The listing builds one solid part. Answer for the finished solid, in the listing's coordinates (mm). A direction names the side the tool comes from. Coordinates: 2 decimals unless noted, no trailing zeros. Order: outer loops, then holes, each group sorted by start corner. A loop starts at its lowest first (then second) coordinate and runs counter-clockwise, first axis right, second up. Notation, with made-up numbers: (78.5, 38.25) -> (108.5, 38.25) arc R20 ccw to (108.5, 59.25) -> close; hole circle Ø3 at (5, -29). An arc over 180 degrees is marked (long way). Return JSON: item names as keys, results as strings.
```python
from build123d import *

# Parameters (mm, degrees)
SKETCH1_W           = 150
SKETCH1_H           = 70
BOSS_EXTRUDE1_DEPTH = 10
SKETCH2_W           = 150
SKETCH2_H           = 3
BOSS_EXTRUDE2_DEPTH = 20
SKETCH3_W           = 110
SKETCH3_H           = 20
CUT_EXTRUDE1_DEPTH  = 105.947605976
FILLET1_R           = 5
FILLET2_R           = 10
FILLET3_R           = 2.5


with BuildPart() as part:
    # Sketch1 → Boss-Extrude1 (new body)
    with BuildSketch(Plane.XY):
        Rectangle(SKETCH1_W, SKETCH1_H)
        Polygon((-60, 25), (-55, 25), (55, 25), (60, 25), (60, 20), (55, 20), (55, -25), (-55, -25), (-55, 20), (-60, 20), align=None, mode=Mode.SUBTRACT)
    extrude(amount=BOSS_EXTRUDE1_DEPTH)

    # Sketch2 → Boss-Extrude2 (add)
    with BuildSketch(Plane.XY.offset(10)):
        with Locations((0, -33.5)):
            Rectangle(SKETCH2_W, SKETCH2_H)
    extrude(amount=BOSS_EXTRUDE2_DEPTH)

    # Sketch3 → Cut-Extrude1 (cut, through all)
    with BuildSketch(Plane(origin=(0, -32, 0), x_dir=(1, 0, 0), z_dir=(0, 1, 0))):
        with Locations((0, -20)):
            Rectangle(SKETCH3_W, SKETCH3_H)
    extrude(amount=-CUT_EXTRUDE1_DEPTH, mode=Mode.SUBTRACT)

    # Fillet1
    fillet1_edges = [part.edges().sort_by_distance(p)[0] for p in [
        (0, 25, 10),
        (0, -25, 10),
        (75, 1.5, 10),
        (0, 35, 10),
        (-75, 1.5, 10),
    ]]
    fillet(fillet1_edges, radius=FILLET1_R - 0.0001)  # a hair under: the kernel refuses the full size

    # Fillet2
    fillet2_edges = [part.edges().sort_by_distance(p)[0] for p in [
        (55, -33.5, 10),
        (-55, -33.5, 10),
    ]]
    fillet(fillet2_edges, radius=FILLET2_R)

    # Fillet3
    fillet3_edges = [part.edges().sort_by_distance(p)[0] for p in [
        (55, -4.99995, 10),
        (-55, -4.99995, 10),
        (-75, -33.5, 30),
        (75, -33.5, 30),
        (55, -33.5, 30),
        (-55, -33.5, 30),
    ]]
    fillet(fillet3_edges, radius=FILLET3_R)


solid = part.part
```
Item 1: Which of the six approach directions +Z, -Z, +X, -X, +Y, -Y give full straight-line access (tool end or side, diameter ignored) to faces 1 (the flat face through (55, -33, 24)), 2 (the flat face through (-1, -31, 0)), 3 (the cylindrical face through (73, 2, 9)), 4 (the flat face through (60, 23, 5)), 5 (the flat face through (-1, 25, 2))?
Answer list:
{"face 1": "+Z, +Y, -Y", "face 2": "-Z, +X, -X, +Y, -Y", "face 3": "+Z, +X, +Y", "face 4": "+Z", "face 5": "+Z, -Z"}
Item 2: Flat-ended cylindrical pins translate along their axes: pin 1 (6 mm diameter, centred on x = -7, z = 13.5, fed in from -Y); pin 2 (8 mm diameter, centred on x = 3, y = -24, fed in from +Z); pin 3 (3 mm diameter, centred on y = 24.5, z = 7.5, fed in from -X); pin 4 (6 mm diameter, centred on y = 15.5, z = 10, fed in from +X). Find the tip coordinate at first contact, or state that the pin passes through.
Answer list:
{"pin 1": "through", "pin 2": "z = 9.58", "pin 3": "x = -74.9", "pin 4": "x = 74.58"}
Item 3: The part is cut by section C-C on z = 15. Determine the outline of the cut face in (x, y).
Answer list:
{"outline": "(-75, -35) -> (-53.66, -35) -> (-53.66, -32) -> (-75, -32) -> close; (53.66, -35) -> (75, -35) -> (75, -32) -> (53.66, -32) -> close"}
Item 4: Find the intervals of material crossed by probe 1 along Y at (x, z) = (47, 2.5); probe 2 along Y at (x, z) = (-61, 12.5); probe 3 along Y at (x, z) = (-41.5, 7.75), in increasing order.
Answer list:
{"probe 1": "-35 to -25, 25 to 35", "probe 2": "-35 to -32", "probe 3": "-35 to -25.82, 25.82 to 34.18"}
Item 5: The part is cut by section D-D on z = 2. Determine the outline of the cut face in (x, y), plus the area to 3 significant figures.
Answer list:
{"outline": "(-75, -35) -> (75, -35) -> (75, 35) -> (-75, 35) -> close; hole (-60, 20) -> (-55, 20) -> (-55, -25) -> (55, -25) -> (55, 20) -> (60, 20) -> (60, 25) -> (-60, 25) -> close", "area": "4,950 mm2"}
Item 6: Determine the mould class of faces 6 (the flat face through (-64, -32, 20)), 7 (the cylindrical face through (-74, 2, 8)), 8 (the cylindrical face through (-1, -27, 9)) for opening direction Y: pulls with the +Y half, pulls with the -Y half, needs draft (parallel to the pull), parting line crosses it, or undercut.
Answer list:
{"face 6": "pulls with the +Y half", "face 7": "needs draft", "face 8": "undercut"}
Item 7: The part is cut by section B-B on y = -10. Determine the outline of the cut face in (x, z).
Answer list:
{"outline": "(-75, 0) -> (-55, 0) -> (-55, 7.5) arc R2.5 ccw to (-57.5, 10) -> (-70, 10) arc R5 ccw to (-75, 5) -> close; (55, 0) -> (75, 0) -> (75, 5) arc R5 ccw to (70, 10) -> (57.5, 10) arc R2.5 ccw to (55, 7.5) -> close"}
